Autodesk Inventor part; units mm, degrees
ref_plane "YZ Plane" through (0, 0, 0) normal (1, 0, 0) x (0, 1, 0)
ref_plane "XZ Plane" through (0, 0, 0) normal (0, 1, 0) x (-1, 0, 0)
ref_plane "XY Plane" through (0, 0, 0) normal (0, 0, 1) x (1, 0, 0)
sketch "スケッチ1" plane through (0, 0, 0) normal (0, 0, 1) x (1, 0, 0)
  line L0 (0, 0) -> (80, 0)
  line L1 (80, 0) -> (80, 50)
  line L2 (40, 0) -> (40, 73.3333) construction
  line L3 (0, 50) -> (0, 0)
  circle A0 centre (10, 10) radius 2.5
  circle A1 centre (70, 10) radius 2.5
  line L4 (10, 10) -> (70, 10) construction
  line L5 (0, 50) -> (80, 50)
  dimension "d2" = 80
  dimension "d6" = 5
  dimension "d7" = 10
  dimension "d14" = 10
  dimension "d17" = 50
extrude "押し出し1" add sketch "スケッチ1" along normal blind 3
properties part number "車軸受け板"
Source: CAD feature listing. Evaluate the final solid. Frame: model axes, mm. Give positions to 0.01 mm unless a question says otherwise; leave off trailing zeros. Write each loop counter-clockwise with the first axis right and the second up, starting at its lowest first coordinate (ties: lowest second). Pieces come first, ordered by that corner, then holes.
1. Section query A-A (x = 70). Return the cut outline in (y, z), then the cut area to 3 significant figures.
2. Material intervals for line 1 along Y through (x, z) = (70, 1.8); line 2 along X through (y, z) = (11, 0.6); line 3 along X through (y, z) = (8.5, 1.85), sorted ascending.
3. Section query B-B (y = 10). Return the cut outline in (x, z).
4. Pull-direction query (Y, two-part tool) for faces 1 (the face through (39, 25, 3)), 2 (the face through (68, 11.5, 1.5)), 3 (the face through (39, 50, 1)); classes: +Y half, -Y half, draft (parallel to the pull), parting line (faces both ways), or undercut.
Output values:
1. outline: (0, 0) - (7.5, 0) - (7.5, 3) - (0, 3) - close; (12.5, 0) - (50, 0) - (50, 3) - (12.5, 3) - close
1. area: 135 mm2
2. line 1: y = 0 to 7.5, 12.5 to 50
2. line 2: x = 0 to 7.71, 12.29 to 67.71, 72.29 to 80
2. line 3: x = 0 to 8, 12 to 68, 72 to 80
3. outline: (0, 0) - (7.5, 0) - (7.5, 3) - (0, 3) - close; (12.5, 0) - (67.5, 0) - (67.5, 3) - (12.5, 3) - close; (72.5, 0) - (80, 0) - (80, 3) - (72.5, 3) - close
4. face 1: draft
4. face 2: undercut
4. face 3: +Y half
